from build123d import *

# Parameters (mm, degrees)
SKETCH_1_R          = 7
EXTRUDE_1_DEPTH     = 15
SKETCH_2_W          = 20
SKETCH_2_H          = 80
EXTRUDE_3_DEPTH     = 120
SKETCH_3_R          = 2.5
SKETCH_3_R_2        = 2
CUT_EXTRUDE_1_DEPTH = 120
SKETCH_4_W          = 102.5
SKETCH_4_H          = 80
EXTRUDE_4_DEPTH     = 40
SKETCH_5_W          = 92.5
SKETCH_5_H          = 80
CUT_EXTRUDE_2_DEPTH = 40
FILLET_1_R          = 10
FILLET_2_RADIUS     = 40
FILLET_2_LENGTH     = 20
FILLET_3_R          = 10
SKETCH_6_R          = 1.75
CUT_EXTRUDE_4_DEPTH = 40
FILLET_5_RADIUS     = 40
FILLET_5_LENGTH     = 15


with BuildPart() as part:
    # 草图1 → 凸台-拉伸1 (new body)
    # profile 1 of 2: a face of its own
    with BuildSketch(Plane(origin=(0, 0, 0), x_dir=(1, 0, 0), z_dir=(0, 1, 0))):
        with BuildLine():
            Line((13, 100), (0, 100))
            Line((0, 100), (0, 60))
            Line((0, 60), (40, 0))
            Line((40, 0), (104, 0))
            Line((104, 0), (144, 60))
            Line((144, 60), (240, 60))
            Line((240, 60), (240, 100))
            Line((240, 100), (153.5, 100))
            ThreePointArc((153.5, 100), (124, 70.5), (94.5, 100))
            Line((94.5, 100), (27, 100))
            ThreePointArc((27, 100), (20, 93), (13, 100))
        make_face()
        with Locations(Location((52, 20, 0), (0, 0, 270))):
            Circle(SKETCH_1_R, mode=Mode.SUBTRACT)
        with Locations(Location((92, 20, 0), (0, 0, 270))):
            Circle(SKETCH_1_R, mode=Mode.SUBTRACT)
    # profile 2 of 2: a face of its own
    with BuildSketch(Plane(origin=(0, 0, 0), x_dir=(1, 0, 0), z_dir=(0, 1, 0))):
        with BuildLine():
            Line((104, 180), (40, 180))
            Line((40, 180), (0, 135.27864045))
            Line((0, 135.27864045), (0, 100))
            Line((0, 100), (13, 100))
            ThreePointArc((13, 100), (20, 107), (27, 100))
            Line((27, 100), (94.5, 100))
            ThreePointArc((94.5, 100), (124, 129.5), (153.5, 100))
            Line((153.5, 100), (240, 100))
            Line((240, 100), (240, 140))
            Line((240, 140), (144, 140))
            Line((144, 140), (104, 180))
        make_face()
    extrude(amount=EXTRUDE_1_DEPTH)

    # 草图2 → 凸台-拉伸3 (add)
    with BuildSketch(Plane(origin=(0, 0, -180), x_dir=(-1, 0, 0), z_dir=(0, 0, -1))):
        with Locations((-50, -25)):
            Rectangle(SKETCH_2_W, SKETCH_2_H)
    extrude(amount=EXTRUDE_3_DEPTH)

    # 草图3 → 切除-拉伸1 (cut)
    with BuildSketch(Plane(origin=(60, 0, 0), x_dir=(0, 0, -1), z_dir=(1, 0, 0))):
        with Locations(Location((240, -25, 0), (0, 0, 90))):
            Circle(SKETCH_3_R)
        with Locations(Location((257.25, -25, 0), (0, 0, 90))):
            Circle(SKETCH_3_R_2)
        with Locations(Location((222.75, -25, 0), (0, 0, 90))):
            Circle(SKETCH_3_R_2)
    extrude(amount=-CUT_EXTRUDE_1_DEPTH, mode=Mode.SUBTRACT)

    # 草图4 → 凸台-拉伸4 (add)
    with BuildSketch(Plane.XZ):
        with Locations((124, -100)):
            Rectangle(SKETCH_4_W, SKETCH_4_H)
    extrude(amount=EXTRUDE_4_DEPTH)

    # 草图5 → 切除-拉伸2 (cut)
    with BuildSketch(Plane.XZ.offset(40)):
        with Locations((124, -100)):
            Rectangle(SKETCH_5_W, SKETCH_5_H)
    extrude(amount=-CUT_EXTRUDE_2_DEPTH, mode=Mode.SUBTRACT)

    # 圆角1
    fillet_1_edges = [part.edges().sort_by_distance(p)[0] for p in [
        (172.75, -40, -140),
        (172.75, -40, -60),
        (75.25, -40, -140),
        (75.25, -40, -60),
    ]]
    fillet(fillet_1_edges, radius=FILLET_1_R)

    # 圆角2: full round fillet: the end face becomes a half cylinder, R = half its width
    fillet_2_face = Plane((50, -25, -300), x_dir=(1, 0, 0), z_dir=(0, 0, -1))  # on the end face: x along it, z out of the body
    fillet_2_slab = fillet_2_face.offset(-FILLET_2_RADIUS / 2) * Box(FILLET_2_LENGTH, 2 * FILLET_2_RADIUS, FILLET_2_RADIUS, mode=Mode.PRIVATE)  # the body's end, R deep
    fillet_2_round = Plane((50, -25, -260), x_dir=(0, 0, -1), z_dir=(1, 0, 0)) * Cylinder(FILLET_2_RADIUS, FILLET_2_LENGTH, mode=Mode.PRIVATE)  # its axis R under the face
    add(fillet_2_slab - fillet_2_round, mode=Mode.SUBTRACT)

    # 圆角3
    fillet_3_edges = [part.edges().sort_by_distance(p)[0] for p in [
        (50, -65, -180),
    ]]
    fillet(fillet_3_edges, radius=FILLET_3_R)

    # 草图6 → 切除-拉伸4 (cut)
    with BuildSketch(Plane(origin=(0, 15, 0), x_dir=(1, 0, 0), z_dir=(0, 1, 0))):
        with Locations(Location((124, 144.5, 0), (0, 0, 270))):
            Circle(SKETCH_6_R)
        with Locations(Location((124, 55.5, 0), (0, 0, 270))):
            Circle(SKETCH_6_R)
    extrude(amount=-CUT_EXTRUDE_4_DEPTH, mode=Mode.SUBTRACT)

    # 圆角5: full round fillet: the end face becomes a half cylinder, R = half its width
    fillet_5_face = Plane((240, 7.5, -100), x_dir=(0, -1, 0), z_dir=(1, 0, 0))  # on the end face: x along it, z out of the body
    fillet_5_slab = fillet_5_face.offset(-FILLET_5_RADIUS / 2) * Box(FILLET_5_LENGTH, 2 * FILLET_5_RADIUS, FILLET_5_RADIUS, mode=Mode.PRIVATE)  # the body's end, R deep
    fillet_5_round = Plane((200, 7.5, -100), x_dir=(1, 0, 0), z_dir=(0, -1, 0)) * Cylinder(FILLET_5_RADIUS, FILLET_5_LENGTH, mode=Mode.PRIVATE)  # its axis R under the face
    add(fillet_5_slab - fillet_5_round, mode=Mode.SUBTRACT)


solid = part.part
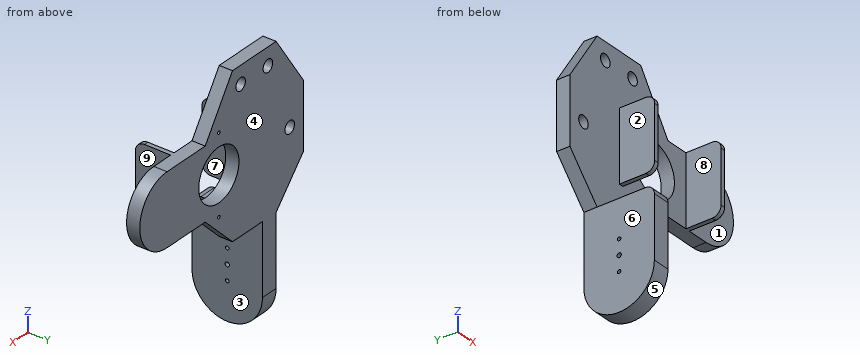
The listing builds one solid part. Answer for the finished solid, in the listing's coordinates (mm). Face numbers are marked on the shaded views. A direction names the side the tool comes from. Coordinates: 2 decimals unless noted, no trailing zeros. Loops run counter-clockwise (first coordinate to the right, second up) from the corner with the lowest first, then second, coordinate; pieces in that order, holes last. Notation, with made-up numbers: M 79.5,88 L 121.5,88 A23 cw 121.5,107 Z; hole C 54.5,-38 d2. An arc over 180 degrees is marked long. Answer in a Markdown table with one row per item.
1) Determine the mould class of the marked faces 6, 7, 8 and 9 for opening direction X: released by +X, released by -X, zero draft, split by the parting line, or undercut.
Answers below:
| item | result |
|---|---|
| face 6 | released by -X |
| face 7 | undercut |
| face 8 | undercut |
| face 9 | released by +X |
2) Which of the six approach directions +Z, -Z, +X, -X, +Y, -Y give full straight-line access (tool end or side, diameter ignored) to the marked faces 1, 2, 3, 4 and 5?
Answers below:
| item | result |
|---|---|
| face 1 | +Z, -Z, +X, -Y |
| face 2 | +Z, -Z, -X, -Y |
| face 3 | -Z, +X, +Y, -Y |
| face 4 | +Z, -Z, +X, -X, +Y |
| face 5 | -Z, +X, -X |
3) Given pin 1 (2 mm diameter, centred on y = -0.5, z = -231, fed in from +X); pin 2 (3 mm diameter, centred on y = -25, z = -240, fed in from -X); pin 3 (7.5 mm diameter, centred on x = 90, y = 9.5, fed in from -Z); pin 4 (5 mm diameter, centred on x = 75.5, y = -12, fed in from +Z), each flat-ended and moving along its own axis, determine where each tip first touches the part or whether it passes through.
Answers below:
| item | result |
|---|---|
| pin 1 | x = 60 |
| pin 2 | through |
| pin 3 | z = -180 |
| pin 4 | z = -60 |
4) Find section A-A (x = 52). Determine the outline of the cut face in (y, z).
Answers below:
| item | result |
|---|---|
| outline | M -65,-260 A40 ccw 15,-260 L 15,-27 L 0,-27 L 0,-180 L -55,-180 A10 ccw -65,-190 Z; M 0,-13 L 15,-13 L 15,0 L 0,0 Z; hole C -25,-240 d5; hole C -25,-257.25 d4; hole C -25,-222.75 d4 |
5) Find section B-B (z = -100). Determine the outline of the cut face in (x, y).
Answers below:
| item | result |
|---|---|
| outline | M 0,0 L 13,0 L 13,15 L 0,15 Z; M 27,0 L 72.75,0 L 72.75,-40 L 77.75,-40 L 77.75,0 L 94.5,0 L 94.5,15 L 27,15 Z; M 153.5,0 L 170.25,0 L 170.25,-40 L 175.25,-40 L 175.25,0 L 240,0 L 240,15 L 153.5,15 Z |
6) Find the intervals of material crossed by probe 1 along X at (y, z) = (-7, -95); probe 2 along Y at (x, z) = (45.25, -257.25); probe 3 along X at (y, z) = (6, -20), in increasing order.
Answers below:
| item | result |
|---|---|
| probe 1 | 72.75 to 77.75, 170.25 to 175.25 |
| probe 2 | -65 to -27, -23 to 15 |
| probe 3 | 26.67 to 45, 59 to 85, 99 to 117.33 |
7) Find section D-D (x = 119). Determine the outline of the cut face in (y, z).
Answers below:
| item | result |
|---|---|
| outline | M 0,-165 L 15,-165 L 15,-129.07 L 0,-129.07 Z; M 0,-70.93 L 15,-70.93 L 15,-22.5 L 0,-22.5 Z |
8) Find section C-C (y = -7.5). Determine the outline of the cut face in (x, z).
Answers below:
| item | result |
|---|---|
| outline | M 40,-295.97 L 60,-295.97 L 60,-180 L 40,-180 Z; M 72.75,-140 L 77.75,-140 L 77.75,-60 L 72.75,-60 Z; M 170.25,-140 L 175.25,-140 L 175.25,-60 L 170.25,-60 Z |
